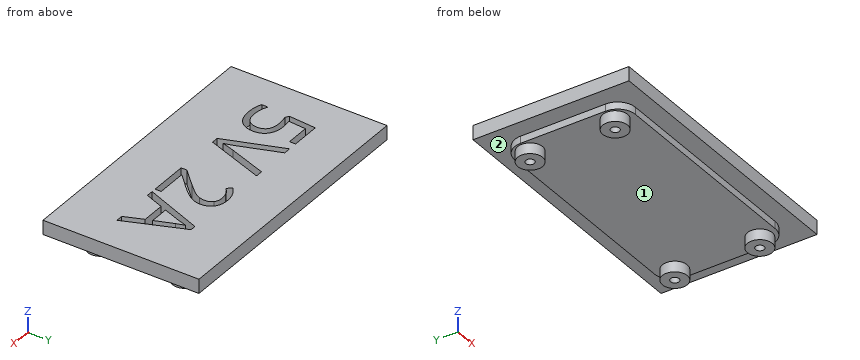
```python
from build123d import *

# Parameters (mm, degrees)
F0_W     = 68
F0_H     = 34
F1_DEPTH = 2
F2_R     = 3.5
F3_DEPTH = 3
F4_D     = 2.4
F4_DEPTH = 3.001
F5_R     = 5
F6_W     = 78
F6_H     = 44
F7_DEPTH = 4


with BuildPart() as f1:
    # F0 (on Top) → F1 (new body)
    with BuildSketch(Plane.XY):
        Rectangle(F0_W, F0_H)
    extrude(amount=F1_DEPTH)

    # F2 (on face) → F3 (join)
    with BuildSketch(Plane.XY):
        with Locations((30, -12)):
            Circle(F2_R)
        with Locations((-30, -12)):
            Circle(F2_R)
        with Locations((30, 12)):
            Circle(F2_R)
        with Locations((-30, 12)):
            Circle(F2_R)
    extrude(amount=-F3_DEPTH)

    # F4 (through all, one way)
    with BuildSketch(Plane.XY):
        with Locations((-30, 12), (-30, -12), (30, 12), (30, -12)):
            Circle(F4_D / 2)
    extrude(amount=-F4_DEPTH, mode=Mode.SUBTRACT)

    # F5
    f5_edges = [f1.edges().sort_by_distance(p)[0] for p in [
        (-34, 17, 1),
        (34, 17, 1),
        (34, -17, 1),
        (-34, -17, 1),
    ]]
    fillet(f5_edges, radius=F5_R)

    # F6 (on face) → F7 (join)
    with BuildSketch(Plane.XY.offset(2)):
        Rectangle(F6_W, F6_H)
        with BuildLine():
            add(Edge.make_bspline(
                [(-27.6022215205, 2.0609542791), (-26.3102811263, 2.3200621019), (-25.0255381717, 2.3200621019)],
                knots=[0, 0, 0, 1, 1, 1], degree=2))
            add(Edge.make_bspline(
                [(-25.0255381717, 2.3200621019), (-22.4272625043, 2.3200621019), (-20.9373925233, 1.0317204275)],
                knots=[0, 0, 0, 1, 1, 1], degree=2))
            add(Edge.make_bspline(
                [(-20.9373925233, 1.0317204275), (-19.4475225423, -0.2566212469), (-19.4475225423, -2.4950249382)],
                knots=[0, 0, 0, 1, 1, 1], degree=2))
            add(Edge.make_bspline(
                [(-19.4475225423, -2.4950249382), (-19.4475225423, -5.0465172487), (-21.0723445143, -6.4986006722)],
                knots=[0, 0, 0, 1, 1, 1], degree=2))
            add(Edge.make_bspline(
                [(-21.0723445143, -6.4986006722), (-22.6971664864, -7.9506840957), (-25.5545499765, -7.9506840957)],
                knots=[0, 0, 0, 1, 1, 1], degree=2))
            add(Edge.make_bspline(
                [(-25.5545499765, -7.9506840957), (-28.3327616319, -7.9506840957), (-29.7938418549, -7.0618003148)],
                knots=[0, 0, 0, 1, 1, 1], degree=2))
            Line((-29.7938418549, -7.0618003148), (-29.7938418549, -5.2624404343))
            add(Edge.make_bspline(
                [(-29.7938418549, -5.2624404343), (-29.009320947, -5.7662612008), (-27.8397370247, -6.0541587817)],
                knots=[0, 0, 0, 1, 1, 1], degree=2))
            add(Edge.make_bspline(
                [(-27.8397370247, -6.0541587817), (-26.6701531024, -6.3420563626), (-25.532957658, -6.3420563626)],
                knots=[0, 0, 0, 1, 1, 1], degree=2))
            add(Edge.make_bspline(
                [(-25.532957658, -6.3420563626), (-23.5536617895, -6.3420563626), (-22.4578516223, -5.4081885846)],
                knots=[0, 0, 0, 1, 1, 1], degree=2))
            add(Edge.make_bspline(
                [(-22.4578516223, -5.4081885846), (-21.3620414551, -4.4743208067), (-21.3620414551, -2.7073494041)],
                knots=[0, 0, 0, 1, 1, 1], degree=2))
            add(Edge.make_bspline(
                [(-21.3620414551, -2.7073494041), (-21.3620414551, 0.7330266874), (-25.5761422951, 0.7330266874)],
                knots=[0, 0, 0, 1, 1, 1], degree=2))
            add(Edge.make_bspline(
                [(-25.5761422951, 0.7330266874), (-26.6449620641, 0.7330266874), (-28.4335257853, 0.4055431891)],
                knots=[0, 0, 0, 1, 1, 1], degree=2))
            Line((-28.4335257853, 0.4055431891), (-29.4015814009, 1.024522988))
            Line((-29.4015814009, 1.024522988), (-28.7826016021, 8.7185858368))
            Line((-28.7826016021, 8.7185858368), (-20.6063103053, 8.7185858368))
            Line((-20.6063103053, 8.7185858368), (-20.6063103053, 6.9983977911))
            Line((-20.6063103053, 6.9983977911), (-27.1847700282, 6.9983977911))
            Line((-27.1847700282, 6.9983977911), (-27.6022215205, 2.0609542791))
        make_face(mode=Mode.SUBTRACT)
        with BuildLine():
            Line((-10.2276025148, -1.8544528207), (-6.4705390845, 8.7185858368))
            Line((-6.4705390845, 8.7185858368), (-4.415670101, 8.7185858368))
            Line((-4.415670101, 8.7185858368), (-10.3391628274, -7.7239647508))
            Line((-10.3391628274, -7.7239647508), (-12.2284907019, -7.7239647508))
            Line((-12.2284907019, -7.7239647508), (-18.1231936703, 8.7185858368))
            Line((-18.1231936703, 8.7185858368), (-16.0971144449, 8.7185858368))
            Line((-16.0971144449, 8.7185858368), (-12.3184586959, -1.9192297764))
            add(Edge.make_bspline(
                [(-12.3184586959, -1.9192297764), (-11.6670904192, -3.7545768545), (-11.2856261245, -5.4855610595)],
                knots=[0, 0, 0, 1, 1, 1], degree=2))
            add(Edge.make_bspline(
                [(-11.2856261245, -5.4855610595), (-10.8789707916, -3.6646088605), (-10.2276025148, -1.8544528207)],
                knots=[0, 0, 0, 1, 1, 1], degree=2))
        make_face(mode=Mode.SUBTRACT)
        with BuildLine():
            Line((13.5023555886, -5.9929805458), (13.5023555886, -7.7239647508))
            Line((13.5023555886, -7.7239647508), (2.6954001466, -7.7239647508))
            Line((2.6954001466, -7.7239647508), (2.6954001466, -6.1153370176))
            Line((2.6954001466, -6.1153370176), (7.0246600189, -1.7644848267))
            add(Edge.make_bspline(
                [(7.0246600189, -1.7644848267), (9.0039558874, 0.2400020801), (9.6337318456, 1.0946980233)],
                knots=[0, 0, 0, 1, 1, 1], degree=2))
            add(Edge.make_bspline(
                [(9.6337318456, 1.0946980233), (10.2635078038, 1.9493939665), (10.5783957828, 2.7591059127)],
                knots=[0, 0, 0, 1, 1, 1], degree=2))
            add(Edge.make_bspline(
                [(10.5783957828, 2.7591059127), (10.8932837619, 3.568817859), (10.8932837619, 4.500886277)],
                knots=[0, 0, 0, 1, 1, 1], degree=2))
            add(Edge.make_bspline(
                [(10.8932837619, 4.500886277), (10.8932837619, 5.8180177095), (10.094367975, 6.5881437384)],
                knots=[0, 0, 0, 1, 1, 1], degree=2))
            add(Edge.make_bspline(
                [(10.094367975, 6.5881437384), (9.2954521881, 7.3582697672), (7.8775566023, 7.3582697672)],
                knots=[0, 0, 0, 1, 1, 1], degree=2))
            add(Edge.make_bspline(
                [(7.8775566023, 7.3582697672), (6.8555201902, 7.3582697672), (5.9378466511, 7.0199901097)],
                knots=[0, 0, 0, 1, 1, 1], degree=2))
            add(Edge.make_bspline(
                [(5.9378466511, 7.0199901097), (5.0201731121, 6.6817104521), (3.8973725467, 5.7928266712)],
                knots=[0, 0, 0, 1, 1, 1], degree=2))
            Line((3.8973725467, 5.7928266712), (2.9077246125, 7.0631747468))
            add(Edge.make_bspline(
                [(2.9077246125, 7.0631747468), (5.1785167816, 8.9525026213), (7.8559642837, 8.9525026213)],
                knots=[0, 0, 0, 1, 1, 1], degree=2))
            add(Edge.make_bspline(
                [(7.8559642837, 8.9525026213), (10.1735398097, 8.9525026213), (11.4888718823, 7.76672446)],
                knots=[0, 0, 0, 1, 1, 1], degree=2))
            add(Edge.make_bspline(
                [(11.4888718823, 7.76672446), (12.804203955, 6.5809462988), (12.804203955, 4.5800581118)],
                knots=[0, 0, 0, 1, 1, 1], degree=2))
            add(Edge.make_bspline(
                [(12.804203955, 4.5800581118), (12.804203955, 3.0146150158), (11.9261163333, 1.4851591174)],
                knots=[0, 0, 0, 1, 1, 1], degree=2))
            add(Edge.make_bspline(
                [(11.9261163333, 1.4851591174), (11.0480287116, -0.044296781), (8.6440839113, -2.3834646256)],
                knots=[0, 0, 0, 1, 1, 1], degree=2))
            Line((8.6440839113, -2.3834646256), (5.0453641504, -5.9030125517))
            Line((5.0453641504, -5.9030125517), (5.0453641504, -5.9929805458))
            Line((5.0453641504, -5.9929805458), (13.5023555886, -5.9929805458))
        make_face(mode=Mode.SUBTRACT)
        Polygon((29.3115314982, -7.7239647508), (27.3322356297, -7.7239647508), (25.2845640858, -2.4950249382), (18.6953082036, -2.4950249382), (16.6728276979, -7.7239647508), (14.7367164666, -7.7239647508), (21.2360043548, 8.7869615123), (22.8446320879, 8.7869615123), align=None, mode=Mode.SUBTRACT)
        with BuildLine():
            Line((19.3718675186, -0.7748368925), (24.6907753252, -0.7748368925))
            Line((24.6907753252, -0.7748368925), (22.7762564124, 4.320950289))
            add(Edge.make_bspline(
                [(22.7762564124, 4.320950289), (22.405588277, 5.2890059047), (22.0133278231, 6.6925066114)],
                knots=[0, 0, 0, 1, 1, 1], degree=2))
            add(Edge.make_bspline(
                [(22.0133278231, 6.6925066114), (21.7650161596, 5.6128906831), (21.3043800302, 4.320950289)],
                knots=[0, 0, 0, 1, 1, 1], degree=2))
            Line((21.3043800302, 4.320950289), (19.3718675186, -0.7748368925))
        make_face()
    extrude(amount=F7_DEPTH)


solid = f1.part
```
Work out the finished part from the listing and answer in its coordinate system (mm). Face numbers are marked on the shaded views. Coordinates: 2 decimals unless noted, no trailing zeros. Loops run counter-clockwise (first coordinate to the right, second up) from the corner with the lowest first, then second, coordinate; pieces in that order, holes last. Notation, with made-up numbers: (-9, 42) -> (4, 42) arc R15 cw to (4, 50) -> close; hole circle Ø9 at (71, -12). An arc over 180 degrees is marked (long way). Answer as CSV lines item,"result".
Q1. The part is cut by section A-A on x = -1.5. Write down the section's boundary in (y, z).
Findings:
outline,"(-22, 2) -> (-17, 2) -> (-17, 0) -> (17, 0) -> (17, 2) -> (22, 2) -> (22, 6) -> (-22, 6) -> close"
Q2. For a pull along X with two mould halves and no side action, classify the marked faces 1 and 2 as +X half, -X half, draft (parallel to the pull), parting line (faces both ways), or undercut.
Findings:
face 1,"undercut"
face 2,"draft"
Q3. The part is cut by section C-C on z = 5. State how many separate pieces and enclosed holes the cut face has, and give its area (3 significant figures).
Findings:
separate pieces,"2"
enclosed holes,"4"
area,"3,180 mm²"
Q4. The part is cut by section B-B on z = 1.25. Write down the section's boundary in (x, y), and give its area (3 significant figures).
Findings:
outline,"(-34, -12) arc R5 ccw to (-29, -17) -> (29, -17) arc R5 ccw to (34, -12) -> (34, 12) arc R5 ccw to (29, 17) -> (-29, 17) arc R5 ccw to (-34, 12) -> close"
area,"2,290 mm²"
Q5. Find the intervals of material crossed by probe 1 along Y at (x, z) = (30, -0.6); probe 2 along Y at (x, z) = (13, 2.25); probe 3 along Z at (x, y) = (-21, -14.5), in increasing order.
Findings:
probe 1,"y = -15.5 to -13.2, -10.8 to -8.5, 8.5 to 10.8, 13.2 to 15.5"
probe 2,"y = -22 to -7.72, -5.99 to 22"
probe 3,"z = 0 to 6"
Q6. Each of these flat-tipped pins is pushed along its axis until it touches: pin 1 (2 mm diameter, centred on x = -30, y = 12, fed in from -Z); pin 2 (0.6 mm diameter, centred on y = 5, z = 1, fed in from -X); pin 3 (1.5 mm diameter, centred on y = 11.5, z = 0.5, fed in from +X). Where does it stop, or does it pass through?
Findings:
pin 1,"stops at z = 0"
pin 2,"stops at x = -34"
pin 3,"stops at x = 34"
